CAD build for the part. Positions are in the model's coordinates, mm. Round coordinates to 2 decimals unless told otherwise and drop trailing zeros. Order: outer loops, then holes, each group sorted by start corner. A loop starts at its lowest first (then second) coordinate and runs counter-clockwise, first axis right, second up. Notation, with made-up numbers: (-37.75, 65) -> (-29.75, 65) arc R28 cw to (-29.75, 92) -> close; hole circle Ø11 at (-30, -18). An arc over 180 degrees is marked (long way). Return JSON: item names as keys, results as strings. Group by question number.
Q1. Mould opens along Z. For faces 1 (the cylindrical face through (1.014, 8.616, -54.385)), 2 (the flat face through (1, 16, -44)), 3 (the flat face through (1, 8, -89)) say: +Z half, -Z half, draft (parallel to the pull), parting line (faces both ways), or undercut.
Q2. Probe line 1 along Z through (x, y) = (1.5, 7.25); line 2 along Z through (x, y) = (1.6, 7); line 3 along Y through (x, z) = (1.3, -31). List the from-to ranges inside material, lowest first.
Q3. Cut at A-A (z = -52). Write the cut outline in (x, y).
Q4. Flat gauge pin, fed straight in: pin 1 (6 mm diameter, centred on y = 4, z = -14.5, fed in from -X). Where does the tip first touch, or does it go through?
Q5. Cut at B-B (x = 0.95). Write the cut outline in (y, z), then the cut area to 3 significant figures.
Autodesk Inventor part; units mm, degrees
ref_plane "YZ Plane" through (0, 0, 0) normal (1, 0, 0) x (0, 1, 0)
ref_plane "XZ Plane" through (0, 0, 0) normal (0, 1, 0) x (-1, 0, 0)
ref_plane "XY Plane" through (0, 0, 0) normal (0, 0, 1) x (1, 0, 0)
sketch "Sketch1" plane through (0, 0, 0) normal (1, 0, 0) x (0, 1, 0)
  line L0 (0, 0) -> (16, 0)
  line L1 (16, 0) -> (16, -89)
  line L2 (16, -89) -> (0, -89)
  line L3 (0, -89) -> (0, 0)
  dimension "d0" = 16
  dimension "d1" = 89
extrude "Extrusion1" add sketch "Sketch1" along normal blind 2
sketch "Sketch2" plane through (2, 0, 0) normal (1, 0, 0) x (0, 0, -1)
  circle A0 centre (76.5, 8.5) radius 1
  circle A1 centre (52, 7.8652) radius 2.5
  circle A2 centre (31, 7.8652) radius 2.5
  circle A3 centre (31, 7.8652) radius 2.5
  circle A4 centre (52, 7.8652) radius 2.5
  circle A5 centre (76.1279, 7.6338) radius 2.5
  line L0 (31, 7.8652) -> (88.1089, 7.8652) construction
  circle A6 centre (76, 7.8652) radius 2.5
  point P0 (0, 0)
  dimension "d4" = 5
  dimension "d5" = 5
  dimension "d6" = 5
  dimension "d9" = 21
  dimension "d10" = 24
extrude "Extrusion2" cut sketch "Sketch2" against normal blind 2 contours A1 | A2 | A6 A5 | A5 A6 picked at (74.9617, 6.4955) picked at (74.7573, 9.9128)
sketch "Sketch3" plane through (2, 8.5, -76.5) normal (1, 0, 0) x (0, 0, -1)
  circle A0 centre (0, 0) radius 1.1582
  point P0 (-76.5, -8.5)
extrude "Extrusion3" cut sketch "Sketch3" against normal blind 10
properties part number "Gear-wall-motor-side"
Solution:
{
 "1": {"face 1": "undercut", "face 2": "draft", "face 3": "-Z half"},
 "2": {"line 1": "z = -89 to -78.42, -73.58 to -54.42, -49.58 to -33.42, -28.58 to 0", "line 2": "z = -89 to -78.35, -73.65 to -54.35, -49.65 to -33.35, -28.65 to 0", "line 3": "y = 0 to 5.37, 10.37 to 16"},
 "3": {"outline": "(0, 0) -> (2, 0) -> (2, 5.37) -> (0, 5.37) -> close; (0, 10.37) -> (2, 10.37) -> (2, 16) -> (0, 16) -> close"},
 "4": {"pin 1": "stops at x = 0"},
 "5": {"outline": "(0, -89) -> (16, -89) -> (16, 0) -> (0, 0) -> close; hole circle Ø5 at (7.87, -76); hole circle Ø5 at (7.87, -52); hole circle Ø5 at (7.87, -31)", "area": "1,370 mm²"}
}
